from build123d import *

# Parameters (mm, degrees)
SKETCH1_R           = 40
BOSS_EXTRUDE1_DEPTH = 80
SKETCH2_R           = 10
CUT_EXTRUDE1_DEPTH  = 50
BOSS_EXTRUDE3_DEPTH = 2
SKETCH7_R           = 10
CUT_EXTRUDE2_DEPTH  = 40
CUT_EXTRUDE3_DEPTH  = 86
BOSS_EXTRUDE5_START = 2
BOSS_EXTRUDE5_DEPTH = 2
SKETCH14_W          = 33.858331452
SKETCH14_H          = 7.7
CUT_EXTRUDE6_DEPTH  = 9


with BuildPart() as part:
    # Sketch1 → Boss-Extrude1 (new body)
    with BuildSketch(Plane.XY):
        Circle(SKETCH1_R)
    extrude(amount=-BOSS_EXTRUDE1_DEPTH)

    # Sketch2 → Cut-Extrude1 (cut)
    with BuildSketch(Plane.XY):
        Circle(SKETCH2_R)
    extrude(amount=-CUT_EXTRUDE1_DEPTH, mode=Mode.SUBTRACT)

    # Sketch5 → Boss-Extrude3 (add)
    with BuildSketch(Plane(origin=(0, 0, -80), x_dir=(-1, 0, 0), z_dir=(0, 0, -1))):
        with BuildLine():
            Line((-2.80604214, 39.953294916), (-2.80604214, 9.637548447))
            ThreePointArc((-2.80604214, 9.637548447), (0.055803254, 10.055803254), (2.917648647, 9.637548447))
            Line((2.917648647, 9.637548447), (2.917648647, 39.953294916))
            ThreePointArc((2.917648647, 39.953294916), (0.055803254, 40.055803254), (-2.80604214, 39.953294916))
        make_face()
        with BuildLine():
            Line((39.953294916, 2.917648647), (9.637548447, 2.917648647))
            ThreePointArc((9.637548447, 2.917648647), (10.055803254, 0.055803254), (9.637548447, -2.80604214))
            Line((9.637548447, -2.80604214), (39.953294916, -2.80604214))
            ThreePointArc((39.953294916, -2.80604214), (40.055803254, 0.055803254), (39.953294916, 2.917648647))
        make_face()
        with BuildLine():
            Line((2.917648647, -39.841688409), (2.917648647, -9.525941939))
            ThreePointArc((2.917648647, -9.525941939), (0.055803254, -9.944196746), (-2.80604214, -9.525941939))
            Line((-2.80604214, -9.525941939), (-2.80604214, -39.841688409))
            ThreePointArc((-2.80604214, -39.841688409), (0.055803254, -39.944196746), (2.917648647, -39.841688409))
        make_face()
        with BuildLine():
            Line((-39.841688409, -2.80604214), (-9.525941939, -2.80604214))
            ThreePointArc((-9.525941939, -2.80604214), (-9.944196746, 0.055803254), (-9.525941939, 2.917648647))
            Line((-9.525941939, 2.917648647), (-39.841688409, 2.917648647))
            ThreePointArc((-39.841688409, 2.917648647), (-39.944196746, 0.055803254), (-39.841688409, -2.80604214))
        make_face()
    extrude(amount=BOSS_EXTRUDE3_DEPTH)

    # Sketch7 → Cut-Extrude2 (cut)
    with BuildSketch(Plane.XY.offset(-50)):
        Circle(SKETCH7_R)
    extrude(amount=-CUT_EXTRUDE2_DEPTH, mode=Mode.SUBTRACT)

    # Sketch10 → Cut-Extrude3 (cut)
    with BuildSketch(Plane.XY):
        with BuildLine():
            ThreePointArc((-9.229165726, -3.85), (-10, 0), (-9.229165726, 3.85))
            Line((-9.229165726, 3.85), (-16.929165726, 3.85))
            Line((-16.929165726, 3.85), (-16.929165726, -3.85))
            Line((-16.929165726, -3.85), (-9.229165726, -3.85))
        make_face()
        with BuildLine():
            Line((16.929165726, 3.85), (9.229165726, 3.85))
            ThreePointArc((9.229165726, 3.85), (9.805397933, 1.963204363), (10, 0))
            ThreePointArc((10, 0), (9.805397933, -1.963204363), (9.229165726, -3.85))
            Line((9.229165726, -3.85), (16.929165726, -3.85))
            Line((16.929165726, -3.85), (16.929165726, 3.85))
        make_face()
    extrude(amount=-CUT_EXTRUDE3_DEPTH, mode=Mode.SUBTRACT)

    # Sketch12 → Boss-Extrude5 (add)
    with BuildSketch(Plane.XY.offset(BOSS_EXTRUDE5_START)):
        with BuildLine():
            Line((-2.61385984, 39.914505342), (-2.61385984, 9.652343588))
            ThreePointArc((-2.61385984, 9.652343588), (0.096784019, 9.898764617), (2.80604214, 9.637548447))
            Line((2.80604214, 9.637548447), (2.61385984, 39.914505342))
            ThreePointArc((2.61385984, 39.914505342), (0, 40), (-2.61385984, 39.914505342))
        make_face()
        with BuildLine():
            Line((39.914505342, 2.61385984), (9.652343588, 2.61385984))
            ThreePointArc((9.652343588, 2.61385984), (9.898764617, -0.096784019), (9.637548447, -2.80604214))
            Line((9.637548447, -2.80604214), (39.914505342, -2.61385984))
            ThreePointArc((39.914505342, -2.61385984), (40, 0), (39.914505342, 2.61385984))
        make_face()
        with BuildLine():
            Line((2.61385984, -39.914505342), (2.61385984, -9.652343588))
            ThreePointArc((2.61385984, -9.652343588), (-0.096784019, -9.898764617), (-2.80604214, -9.637548447))
            Line((-2.80604214, -9.637548447), (-2.61385984, -39.914505342))
            ThreePointArc((-2.61385984, -39.914505342), (0, -40), (2.61385984, -39.914505342))
        make_face()
        with BuildLine():
            Line((-39.914505342, -2.61385984), (-9.652343588, -2.61385984))
            ThreePointArc((-9.652343588, -2.61385984), (-9.898764617, 0.096784019), (-9.637548447, 2.80604214))
            Line((-9.637548447, 2.80604214), (-39.914505342, 2.61385984))
            ThreePointArc((-39.914505342, 2.61385984), (-40, 0), (-39.914505342, -2.61385984))
        make_face()
    extrude(amount=-BOSS_EXTRUDE5_DEPTH)

    # Sketch14 → Cut-Extrude6 (cut)
    with BuildSketch(Plane.XY.offset(2)):
        Rectangle(SKETCH14_W, SKETCH14_H)
    extrude(amount=-CUT_EXTRUDE6_DEPTH, mode=Mode.SUBTRACT)


solid = part.part
Input: part model. Units: mm. Frame: model coordinates. A direction names the side the tool comes from. Coordinates: 2 decimals unless noted, no trailing zeros. Loops run counter-clockwise (first coordinate to the right, second up) from the corner with the lowest first, then second, coordinate; pieces in that order, holes last. Notation, with made-up numbers: (78, 39.25) -> (130, 39.25) arc R33 ccw to (130, 75.25) -> close; hole circle Ø11 at (45, 46). An arc over 180 degrees is marked (long way). Write each question's results on one line, items separated by ' | '. Start each with the question number.
Q1. Section D-D, the plane y = -17. Return the cut outline in (x, z), plus the area to 3 significant figures.
Q2. Pin query (flat end, axial travel): pin 1 (1 mm diameter, centred on x = 28.5, z = -81, fed in from +Y); pin 2 (10 mm diameter, centred on x = -18.5, z = -70, fed in from -Y); pin 3 (1 mm diameter, centred on x = -25, z = -81, fed in from -Y). Return the tip coordinate at first contact, or that it passes through.
Q3. Section A-A, the plane x = 0. Return the cut outline in (y, z).
Q4. Section C-C, the plane x = -19. Return the cut outline in (y, z), plus the area to 3 significant figures.
Q5. Reachability of faces 3 (the flat face through (17, 17, 0)), 4 (the flat face through (-17, -17, 0)), 5 (the flat face through (13, 3.85, -39)), 6 (the flat face through (17, -17, 0)) from +Z, -Z, +X, -X, +Y, -Y: full face, straight path, thin tool, end or side. Return the list, or none.
Q6. Ray query, line 1 (X direction, y = 1, z = -52.5); line 2 (X direction, y = 2.5, z = -18); line 3 (Z direction, x = 14, y = -33). Return the intervals inside material, ascending. Write a range as from..to.
Q7. Pull-direction query (X, two-part tool) for faces 1 (the cylindrical face through (0, -10, -40)), 2 (the flat face through (0, -25, -82)); classes: released by +X, released by -X, zero draft, split by the parting line, or undercut.
Q8. Section B-B, the plane y = 0. Return the cut outline in (x, z).
Found:
1) outline: (-36.21, -80) -> (-2.92, -80) -> (-2.92, -82) -> (2.81, -82) -> (2.81, -80) -> (36.21, -80) -> (36.21, 0) -> (2.61, 0) -> (2.61, 2) -> (-2.76, 2) -> (-2.76, 0) -> (-36.21, 0) -> close | area: 5,820 mm2
2) pin 1: y = 2.92 | pin 2: y = -37.65 | pin 3: y = -2.81
3) outline: (-40, -80) -> (-39.94, -80) -> (-39.94, -82) -> (-10, -82) -> (-10, 0) -> (-9.9, 0) -> (-9.9, 2) -> (-40, 2) -> close; (9.9, 0) -> (10, 0) -> (10, -80) -> (10.06, -80) -> (10.06, -82) -> (40.06, -82) -> (40.06, -80) -> (40, -80) -> (40, 2) -> (9.9, 2) -> close
4) outline: (-35.2, -80) -> (-2.81, -80) -> (-2.81, -82) -> (2.92, -82) -> (2.92, -80) -> (35.2, -80) -> (35.2, 0) -> (2.75, 0) -> (2.75, 2) -> (-2.61, 2) -> (-2.61, 0) -> (-35.2, 0) -> close | area: 5,650 mm2
5) face 3: +Z, +X, +Y | face 4: +Z, -X, -Y | face 5: +Z, -Z | face 6: +Z, +X, -Y
6) line 1: -39.99..-16.93, 16.93..39.99 | line 2: -39.92..-16.93, 16.93..39.92 | line 3: -80..0
7) face 1: undercut | face 2: zero draft
8) outline: (-40.06, -82) -> (-16.93, -82) -> (-16.93, 2) -> (-40, 2) -> (-40, -80) -> (-40.06, -80) -> close; (16.93, -82) -> (39.94, -82) -> (39.94, -80) -> (40, -80) -> (40, 2) -> (16.93, 2) -> close
